```python
from build123d import *

# Parameters (mm, degrees)
EXTRUDE1_DEPTH                   = 1.25
CUT_EXTRUDE4_DEPTH               = 3.5
FURO_COM_FOLGA_DE_M31_AT_2_COUNT = 2
FURO_COM_FOLGA_DE_M31_AT_2_PITCH = 100
FURO_COM_FOLGA_DE_M31_AT_3_COUNT = 2
FURO_COM_FOLGA_DE_M31_AT_3_PITCH = 100
FURO_COM_FOLGA_DE_M31_AT_4_COUNT = 2
FURO_COM_FOLGA_DE_M31_AT_4_PITCH = 157.608692654
FURO_COM_FOLGA_DE_M31_AT_5_COUNT = 2
FURO_COM_FOLGA_DE_M31_AT_5_PITCH = 157.608692654


with BuildPart() as part:
    # Sketch1 → Extrude1 (new body, symmetric)
    with BuildSketch(Plane.XY):
        with BuildLine():
            Line((-144.5, 92.5), (144.5, 92.5))
            ThreePointArc((144.5, 92.5), (146.621320344, 91.621320344), (147.5, 89.5))
            Line((147.5, 89.5), (147.5, -89.5))
            ThreePointArc((147.5, -89.5), (146.621320344, -91.621320344), (144.5, -92.5))
            Line((144.5, -92.5), (-144.5, -92.5))
            ThreePointArc((-144.5, -92.5), (-146.621320344, -91.621320344), (-147.5, -89.5))
            Line((-147.5, -89.5), (-147.5, 89.5))
            ThreePointArc((-147.5, 89.5), (-146.621320344, 91.621320344), (-144.5, 92.5))
        make_face()
    extrude(amount=EXTRUDE1_DEPTH, both=True)

    # Sketch5 → Cut-Extrude4 (cut, through all)
    with BuildSketch(Plane.XY.offset(1.25)):
        with BuildLine():
            Line((-127, 74.5), (127, 74.5))
            ThreePointArc((127, 74.5), (128.767766953, 73.767766953), (129.5, 72))
            Line((129.5, 72), (129.5, -72))
            ThreePointArc((129.5, -72), (128.767766953, -73.767766953), (127, -74.5))
            Line((127, -74.5), (-127, -74.5))
            ThreePointArc((-127, -74.5), (-128.767766953, -73.767766953), (-129.5, -72))
            Line((-129.5, -72), (-129.5, 72))
            ThreePointArc((-129.5, 72), (-128.767766953, 73.767766953), (-127, 74.5))
        make_face()
    extrude(amount=-CUT_EXTRUDE4_DEPTH, mode=Mode.SUBTRACT)

    # Esboço1 → Escareado para SFHCS M41 (revolve, cut)
    with BuildSketch(Plane(origin=(139, 83.5, 1.25), x_dir=(0, -1, 0), z_dir=(1, 0, 0))):
        Polygon((0, 0), (0, 2.5), (2.25, 2.5), (2.25, 2.23), (4.48, 0), align=None)
    escareado_para_sfhcs_m41 = revolve(axis=Axis((139, 83.5, 7.6), (0, 0, -1)), mode=Mode.SUBTRACT)

    # Esboço3 → Furo com folga de M31 (revolve, cut)
    with BuildSketch(Plane(origin=(0, -80.5, 1.25), x_dir=(0, -1, 0), z_dir=(1, 0, 0))):
        Polygon((0, 0), (0, 2.5), (1.7, 2.5), (1.7, 1.3), (3, 0), align=None)
    furo_com_folga_de_m31 = revolve(axis=Axis((0, -80.5, 7.6), (0, 0, -1)), mode=Mode.SUBTRACT)

    # Furo com folga de M31 at 2: Furo com folga de M31 ×2
    with Locations(*[(-i * FURO_COM_FOLGA_DE_M31_AT_2_PITCH, 0, 0) for i in range(1, FURO_COM_FOLGA_DE_M31_AT_2_COUNT)]):
        add(furo_com_folga_de_m31, mode=Mode.SUBTRACT)

    # Furo com folga de M31 at 3: Furo com folga de M31 ×2
    with Locations(*[(i * FURO_COM_FOLGA_DE_M31_AT_3_PITCH, 0, 0) for i in range(1, FURO_COM_FOLGA_DE_M31_AT_3_COUNT)]):
        add(furo_com_folga_de_m31, mode=Mode.SUBTRACT)

    # Furo com folga de M31 at 4: Furo com folga de M31 ×2
    with Locations(*[Vector(-0.859724154, 0.51075863, 0) * (i * FURO_COM_FOLGA_DE_M31_AT_4_PITCH) for i in range(1, FURO_COM_FOLGA_DE_M31_AT_4_COUNT)]):
        add(furo_com_folga_de_m31, mode=Mode.SUBTRACT)

    # Furo com folga de M31 at 5: Furo com folga de M31 ×2
    with Locations(*[Vector(0.859724154, 0.51075863, 0) * (i * FURO_COM_FOLGA_DE_M31_AT_5_PITCH) for i in range(1, FURO_COM_FOLGA_DE_M31_AT_5_COUNT)]):
        add(furo_com_folga_de_m31, mode=Mode.SUBTRACT)

    # Espelhar1: Furo com folga de M31 across plane
    add(furo_com_folga_de_m31.mirror(Plane.ZX), mode=Mode.SUBTRACT)

    # Espelhar1 copy 1 sketch → Espelhar1 copy 1 (revolve, cut)
    with BuildSketch(Plane(origin=(-100, 80.5, 1.25), x_dir=(0, 1, 0), z_dir=(1, 0, 0))):
        Polygon((0, 0), (0, -2.5), (1.7, -2.5), (1.7, -1.3), (3, 0), align=None)
    revolve(axis=Axis((-100, 80.5, 7.6), (0, 0, 1)), mode=Mode.SUBTRACT)

    # Espelhar1 copy 2 sketch → Espelhar1 copy 2 (revolve, cut)
    with BuildSketch(Plane(origin=(100, 80.5, 1.25), x_dir=(0, 1, 0), z_dir=(1, 0, 0))):
        Polygon((0, 0), (0, -2.5), (1.7, -2.5), (1.7, -1.3), (3, 0), align=None)
    revolve(axis=Axis((100, 80.5, 7.6), (0, 0, 1)), mode=Mode.SUBTRACT)

    # Espelhar1 copy 3 sketch → Espelhar1 copy 3 (revolve, cut)
    with BuildSketch(Plane(origin=(-135.5, 0, 1.25), x_dir=(0, 1, 0), z_dir=(1, 0, 0))):
        Polygon((0, 0), (0, -2.5), (1.7, -2.5), (1.7, -1.3), (3, 0), align=None)
    revolve(axis=Axis((-135.5, 0, 7.6), (0, 0, 1)), mode=Mode.SUBTRACT)

    # Espelhar1 copy 4 sketch → Espelhar1 copy 4 (revolve, cut)
    with BuildSketch(Plane(origin=(135.5, 0, 1.25), x_dir=(0, 1, 0), z_dir=(1, 0, 0))):
        Polygon((0, 0), (0, -2.5), (1.7, -2.5), (1.7, -1.3), (3, 0), align=None)
    revolve(axis=Axis((135.5, 0, 7.6), (0, 0, 1)), mode=Mode.SUBTRACT)

    # Espelhar2: Escareado para SFHCS M41 across plane
    add(escareado_para_sfhcs_m41.mirror(Plane(origin=(0, 0, 0), x_dir=(0, 0, 1), z_dir=(1, 0, 0))), mode=Mode.SUBTRACT)

    # Espelhar3: Escareado para SFHCS M41 across plane
    add(escareado_para_sfhcs_m41.mirror(Plane.ZX), mode=Mode.SUBTRACT)

    # Espelhar3 copy 1 sketch → Espelhar3 copy 1 (revolve, cut)
    with BuildSketch(Plane(origin=(-139, -83.5, 1.25), x_dir=(0, 1, 0), z_dir=(-1, 0, 0))):
        Polygon((0, 0), (0, 2.5), (2.25, 2.5), (2.25, 2.23), (4.48, 0), align=None)
    revolve(axis=Axis((-139, -83.5, 7.6), (0, 0, -1)), mode=Mode.SUBTRACT)


solid = part.part
```
Verification items for the finished model (mm, model axes). Give positions to 0.01 mm unless a question says otherwise; leave off trailing zeros. Loops run counter-clockwise (first coordinate to the right, second up) from the corner with the lowest first, then second, coordinate; pieces in that order, holes last.
1. Section check C-C, the plane x = 94. Enter the section's corners in (y, z).
2. Mould release check, pull along X, two halves, no side actions. Record for faces 1 (the flat face through (23, -75, 1.25)), 2 (the conical face through (-141.33, 84.02, -0.84)), 3 (the conical face through (141.33, -84.02, -0.84)): released by +X, released by -X, zero draft, split by the parting line, or undercut.
3. Section check B-B, the plane z = -0.45. Count the separate pieces of the cut face and the enclosed holes in it, then the cut area to 3 significant figures.
4. Section check A-A, the plane y = -28. Enter the section's corners in (x, z), then the cut area to 3 significant figures.
5. Go/stop test with flat-tipped pins: pin 1 Ø6 at (x, y) = (-139, -83.5) entering from +Z; pin 2 Ø5 at (x, y) = (139, -83.5) entering from +Z; pin 3 Ø2.5 at (x, y) = (-135.5, 0) entering from -Z. Record where each tip stops, or that it passes through.
6. Thickness scan on line 1 (Y direction, x = 100, z = -0.4); line 2 (X direction, y = -80.5, z = -0.6); line 3 (X direction, y = 0, z = -0.7). Record the ranges inside material, lowest first.
Geometry says:
1. outline: (-92.5, -1.25) - (-74.5, -1.25) - (-74.5, 1.25) - (-92.5, 1.25) - close; (74.5, -1.25) - (92.5, -1.25) - (92.5, 1.25) - (74.5, 1.25) - close
2. face 1: zero draft
2. face 2: undercut
2. face 3: undercut
3. separate pieces: 1
3. enclosed holes: 13
3. area: 15,800 mm2
4. outline: (-147.5, -1.25) - (-129.5, -1.25) - (-129.5, 1.25) - (-147.5, 1.25) - close; (129.5, -1.25) - (147.5, -1.25) - (147.5, 1.25) - (129.5, 1.25) - close
4. area: 90.0 mm2
5. pin 1: stops at z = -0.23
5. pin 2: stops at z = -0.73
5. pin 3: passes through
6. line 1: y = -92.5 to -82.2, -78.8 to -74.5, 74.5 to 78.8, 82.2 to 92.5
6. line 2: x = -147.5 to -101.7, -98.3 to -1.7, 1.7 to 98.3, 101.7 to 147.5
6. line 3: x = -147.5 to -137.2, -133.8 to -129.5, 129.5 to 133.8, 137.2 to 147.5
